Here's how the part is built. I have some questions about the finished solid (model axes, mm). A direction names the side the tool comes from. Give positions to 0.01 mm unless a question says otherwise; leave off trailing zeros. Write each loop counter-clockwise with the first axis right and the second up, starting at its lowest first coordinate (ties: lowest second). Pieces come first, ordered by that corner, then holes. Notation, with made-up numbers: (87.25, 57.5) -> (139.25, 57.5) arc R10 cw to (139.25, 67.5) -> close; hole circle Ø11 at (47.25, 71). An arc over 180 degrees is marked (long way). Use CSV: the item, a comma, the result in double quotes. Start each with the question number.
(1) If we mould it in two halves opening along Y, with no side actions, what happens to faces 5 (the flat face through (157, 0, 2)), 6 (the flat face through (183, -195, 2)), 7 (the flat face through (115, 0, 3)), 8 (the cylindrical face through (-1.5, -32.8, 2.5))? For each: pulls with the +Y half, pulls with the -Y half, needs draft (parallel to the pull), parting line crosses it, or undercut.
(2) Suppose I cut it at C-C on z = 3.4. Give the number of separate pieces and of enclosed holes in the cut face, plus the area to 3 significant figures.
(3) Suppose I cut it at D-D on y = -105. List the corners of the cut face in (x, z) for me, plus the area to 3 significant figures.
(4) I need wall thicknesses on L1, parallel to Y at x = 103, z = 1.7; L2, parallel to Y at x = 2.5, z = 3.15; L3, parallel to Y at x = 177.9, z = 2.65. Which ranges of each line are inside material? Lowest first, please. Write a range as [from, to].
(5) Suppose I cut it at A-A on x = 118. List the corners of the cut face in (y, z) for me.
(6) Suppose I cut it at B-B on x = 47.5. List the corners of the cut face in (y, z) for me.
(7) For pin 1 Ø2.5 at (y, z) = (-2, 3) entering from -X; pin 2 Ø2 at (y, z) = (-127.5, 3) entering from +X; pin 3 Ø2.5 at (x, z) = (115, 2.5) entering from +Y, each with a flat end and sliding along its axis, tell me the tip position at first contact or that it passes through.
(8) Which directions (+Z, -Z, +X, -X, +Y, -Y) give clear straight access to the entire face, cutting with the end or side of a thin tool? Please do faces 1 (the flat face through (0, -48, 2)), 2 (the flat face through (23, -190, 3)), 3 (the flat face through (113.7, -163, 3)), 4 (the flat face through (192, -48, 2)).
from build123d import *

# Parameters (mm, degrees)
SKETCH1_R           = 2.1
BOSS_EXTRUDE1_DEPTH = 5
SKETCH5_W           = 35
SKETCH5_H           = 5
SKETCH5_W_2         = 10
CUT_EXTRUDE2_DEPTH  = 5
SKETCH6_R           = 2.1
CUT_EXTRUDE3_DEPTH  = 5
SKETCH8_R           = 2.1
SKETCH8_W           = 10
SKETCH8_H           = 5
CUT_EXTRUDE4_DEPTH  = 5
BOSS_EXTRUDE3_START = -5
BOSS_EXTRUDE3_DEPTH = 5
SKETCH12_W          = 10.4
SKETCH12_H          = 5
CUT_EXTRUDE5_DEPTH  = 5
SKETCH13_W          = 35.4
SKETCH13_H          = 5.4
CUT_EXTRUDE6_DEPTH  = 5
SKETCH16_W          = 50
SKETCH16_H          = 60.4
CUT_EXTRUDE8_DEPTH  = 5
SKETCH17_W          = 6.8
SKETCH17_H          = 4.2
SKETCH17_W_2        = 3.2
SKETCH17_H_2        = 1.4
SKETCH17_W_3        = 7
CUT_EXTRUDE9_DEPTH  = 5


with BuildPart() as part:
    # Sketch1 → Boss-Extrude1 (new body)
    with BuildSketch(Plane.XY):
        with BuildLine():
            ThreePointArc((0, -29.777501001), (-1.5, -32.9), (0, -36.022498999))
            Line((0, -36.022498999), (0, -60))
            Line((0, -60), (50, -60))
            Line((50, -60), (50, -120))
            Line((50, -120), (0, -120))
            Line((0, -120), (0, -131.177501001))
            ThreePointArc((0, -131.177501001), (-1.5, -134.3), (0, -137.422498999))
            Line((0, -137.422498999), (0, -195))
            Line((0, -195), (192, -195))
            Line((192, -195), (192, -137.422498999))
            ThreePointArc((192, -137.422498999), (193.5, -134.3), (192, -131.177501001))
            Line((192, -131.177501001), (192, -120))
            Line((192, -120), (142, -120))
            Line((142, -120), (142, -60))
            Line((142, -60), (192, -60))
            Line((192, -60), (192, -36.022498999))
            ThreePointArc((192, -36.022498999), (193.5, -32.9), (192, -29.777501001))
            Line((192, -29.777501001), (192, 0))
            Line((192, 0), (122, 0))
            Line((122, 0), (122, 5))
            Line((122, 5), (99.122498999, 5))
            ThreePointArc((99.122498999, 5), (96, 6.5), (92.877501001, 5))
            Line((92.877501001, 5), (70, 5))
            Line((70, 5), (70, 0))
            Line((70, 0), (59, 0))
            Line((59, 0), (0, 0))
            Line((0, 0), (0, -21))
            Line((0, -21), (0, -29.777501001))
        make_face()
        with Locations((2.5, -134.3)):
            Circle(SKETCH1_R, mode=Mode.SUBTRACT)
        with Locations((189.5, -134.3)):
            Circle(SKETCH1_R, mode=Mode.SUBTRACT)
        with Locations((2.5, -32.9)):
            Circle(SKETCH1_R, mode=Mode.SUBTRACT)
        with Locations((96, 2.5)):
            Circle(SKETCH1_R, mode=Mode.SUBTRACT)
        with Locations((189.5, -32.9)):
            Circle(SKETCH1_R, mode=Mode.SUBTRACT)
    extrude(amount=BOSS_EXTRUDE1_DEPTH)

    # Sketch5 → Cut-Extrude2 (cut)
    with BuildSketch(Plane.XY.offset(5)):
        with Locations((96, -163.217967697)):
            Rectangle(SKETCH5_W, SKETCH5_H)
        with Locations((96, -120)):
            Rectangle(SKETCH5_W, SKETCH5_H)
        with Locations((23, -192.5)):
            Rectangle(SKETCH5_W_2, SKETCH5_H)
        with Locations((169, -192.5)):
            Rectangle(SKETCH5_W_2, SKETCH5_H)
    extrude(amount=-CUT_EXTRUDE2_DEPTH, mode=Mode.SUBTRACT)

    # Sketch6 → Cut-Extrude3 (cut)
    with BuildSketch(Plane.XY.offset(5)):
        with Locations((213.012247999, -33.340051313)):
            Circle(SKETCH6_R)
        with Locations((177.9, -192.5)):
            Circle(SKETCH6_R)
        with Locations(Location((160.1, -192.5, 0), (0, 0, 180))):
            Circle(SKETCH6_R)
        with Locations((-21.012247999, -33.340051313)):
            Circle(SKETCH6_R)
        with Locations((31.9, -192.5)):
            Circle(SKETCH6_R)
        with Locations(Location((14.1, -192.5, 0), (0, 0, 180))):
            Circle(SKETCH6_R)
        with Locations((126, -120)):
            Circle(SKETCH6_R)
        with Locations((126, -163.217967697)):
            Circle(SKETCH6_R)
        with Locations(Location((66, -163.217967697, 0), (0, 0, 180))):
            Circle(SKETCH6_R)
        with Locations(Location((66, -120, 0), (0, 0, 180))):
            Circle(SKETCH6_R)
    extrude(amount=-CUT_EXTRUDE3_DEPTH, mode=Mode.SUBTRACT)

    # Sketch8 → Cut-Extrude4 (cut)
    with BuildSketch(Plane.XY.offset(5)):
        with Locations((88.012247999, -2.5)):
            Circle(SKETCH8_R)
        with Locations((103.012247999, -2.5)):
            Circle(SKETCH8_R)
        with Locations((75.512247999, -2.5)):
            Rectangle(SKETCH8_W, SKETCH8_H)
        with Locations((115.512247999, -2.5)):
            Rectangle(SKETCH8_W, SKETCH8_H)
    extrude(amount=-CUT_EXTRUDE4_DEPTH, mode=Mode.SUBTRACT)

    # Sketch9 → Boss-Extrude3 (add)
    with BuildSketch(Plane.XY.offset(5).offset(BOSS_EXTRUDE3_START)):
        with BuildLine():
            Line((-19, -130), (0, -130))
            Line((0, -130), (0, -131.177501001))
            ThreePointArc((0, -131.177501001), (-1.5, -134.3), (0, -137.422498999))
            Line((0, -137.422498999), (0, -153))
            Line((0, -153), (-19, -153))
            Line((-19, -153), (-19, -130))
        make_face()
    boss_extrude3 = extrude(amount=BOSS_EXTRUDE3_DEPTH)

    # Sketch12 → Cut-Extrude5 (cut)
    with BuildSketch(Plane.XY.offset(5)):
        with Locations((23, -192.5)):
            Rectangle(SKETCH12_W, SKETCH12_H)
        with Locations((169, -192.5)):
            Rectangle(SKETCH12_W, SKETCH12_H)
    extrude(amount=-CUT_EXTRUDE5_DEPTH, mode=Mode.SUBTRACT)

    # Sketch13 → Cut-Extrude6 (cut)
    with BuildSketch(Plane.XY.offset(5)):
        with Locations((96, -120)):
            Rectangle(SKETCH13_W, SKETCH13_H)
        with Locations((96, -163.217967697)):
            Rectangle(SKETCH13_W, SKETCH13_H)
    extrude(amount=-CUT_EXTRUDE6_DEPTH, mode=Mode.SUBTRACT)

    # Sketch16 → Cut-Extrude8 (cut)
    with BuildSketch(Plane.XY.offset(5)):
        with Locations((25, -90)):
            Rectangle(SKETCH16_W, SKETCH16_H)
        with Locations((167, -90)):
            Rectangle(SKETCH16_W, SKETCH16_H)
    extrude(amount=-CUT_EXTRUDE8_DEPTH, mode=Mode.SUBTRACT)

    # Mirror2: Boss-Extrude3 across plane
    add(boss_extrude3.mirror(Plane(origin=(96, 0, 0), x_dir=(0, 0, 1), z_dir=(1, 0, 0))))

    # Sketch17 → Cut-Extrude9 (cut)
    with BuildSketch(Plane.XY.offset(5)):
        with Locations((207.6, -141.5)):
            Rectangle(SKETCH17_W, SKETCH17_H)
        with Locations((202.6, -141.5)):
            Rectangle(SKETCH17_W_2, SKETCH17_H)
        with Locations((202.6, -138.7)):
            Rectangle(SKETCH17_W_2, SKETCH17_H_2)
        with Locations((197.5, -141.5)):
            Rectangle(SKETCH17_W_3, SKETCH17_H)
        with Locations((202.6, -144.3)):
            Rectangle(SKETCH17_W_2, SKETCH17_H_2)
        with Locations((-15.6, -141.5)):
            Rectangle(SKETCH17_W, SKETCH17_H)
        with Locations((-10.6, -138.7)):
            Rectangle(SKETCH17_W_2, SKETCH17_H_2)
        with Locations((-10.6, -141.5)):
            Rectangle(SKETCH17_W_2, SKETCH17_H)
        with Locations((-5.5, -141.5)):
            Rectangle(SKETCH17_W_3, SKETCH17_H)
        with Locations((-10.6, -144.3)):
            Rectangle(SKETCH17_W_2, SKETCH17_H_2)
    extrude(amount=-CUT_EXTRUDE9_DEPTH, mode=Mode.SUBTRACT)


solid = part.part
Geometry says:
1,face 5,"pulls with the +Y half"
1,face 6,"pulls with the -Y half"
1,face 7,"undercut"
1,face 8,"undercut"
2,separate pieces,"1"
2,enclosed holes,"19"
2,area,"31,600 mm²"
3,outline,"(50, 0) -> (142, 0) -> (142, 5) -> (50, 5) -> close"
3,area,"460 mm²"
4,L1,"[-195, -165.92], [-160.52, -122.7], [-117.3, -4.6], [-0.4, 5]"
4,L2,"[-195, -136.4], [-132.2, -120.2], [-59.8, -35], [-30.8, 0]"
4,L3,"[-195, -194.6], [-190.4, -120.2], [-59.8, 0]"
5,outline,"(-195, 0) -> (-5, 0) -> (-5, 5) -> (-195, 5) -> close; (0, 0) -> (5, 0) -> (5, 5) -> (0, 5) -> close"
6,outline,"(-195, 0) -> (-120.2, 0) -> (-120.2, 5) -> (-195, 5) -> close; (-59.8, 0) -> (0, 0) -> (0, 5) -> (-59.8, 5) -> close"
7,pin 1,"x = 0"
7,pin 2,"x = 192"
7,pin 3,"y = 5"
8,face 1,"+Z, -Z, -X"
8,face 2,"+Z, -Z, -Y"
8,face 3,"+Z, -Z"
8,face 4,"+Z, -Z, +X"
